from build123d import *

# Parameters (mm, degrees)
CYLINDER002_R     = 35
CYLINDER002_DEPTH = 50
CYLINDER001_R     = 35
CYLINDER001_DEPTH = 50
BOX001_W          = 102
BOX001_H          = 260
BOX001_DEPTH      = 50
CYLINDER_R        = 37
CYLINDER_DEPTH    = 45
CYLINDER003_R     = 37
CYLINDER003_DEPTH = 45
BOX_W             = 40
BOX_H             = 270
BOX_DEPTH         = 25
CHAMFER_SIZE      = 1.5


with BuildPart() as cylinder002:
    # Cylinder002 → Cylinder002 (new body)
    with BuildSketch(Plane(origin=(40, 230, -45), x_dir=(1, 0, 0), z_dir=(0, 0, 1))):
        Circle(CYLINDER002_R)
    extrude(amount=CYLINDER002_DEPTH)


with BuildPart() as cylinder001:
    # Cylinder001 → Cylinder001 (new body)
    with BuildSketch(Plane(origin=(40, 40, -45), x_dir=(1, 0, 0), z_dir=(0, 0, 1))):
        Circle(CYLINDER001_R)
    extrude(amount=CYLINDER001_DEPTH)


with BuildPart() as main_cutout:
    # Box001 → Box001 (new body)
    with BuildSketch(Plane(origin=(5, 5, 5), x_dir=(1, 0, 0), z_dir=(0, 0, 1))):
        with Locations((51, 130)):
            Rectangle(BOX001_W, BOX001_H)
    extrude(amount=BOX001_DEPTH)


with BuildPart() as cylinder:
    # Cylinder → Cylinder (new body)
    with BuildSketch(Plane(origin=(40, 40, -20), x_dir=(1, 0, 0), z_dir=(0, 0, 1))):
        Circle(CYLINDER_R)
    extrude(amount=CYLINDER_DEPTH)


with BuildPart() as cylinder003:
    # Cylinder003 → Cylinder003 (new body)
    with BuildSketch(Plane(origin=(40, 230, -20), x_dir=(1, 0, 0), z_dir=(0, 0, 1))):
        Circle(CYLINDER003_R)
    extrude(amount=CYLINDER003_DEPTH)


with BuildPart() as chamfer_body:
    # Box → Box (new body)
    with BuildSketch(Plane.XY):
        with Locations((20, 135)):
            Rectangle(BOX_W, BOX_H)
    extrude(amount=BOX_DEPTH)

    # Fusion: union Cylinder, Cylinder003
    add(cylinder.part)
    add(cylinder003.part)

    # Cut: cut Main cutout
    add(main_cutout.part, mode=Mode.SUBTRACT)

    # Cut001: cut Cylinder001
    add(cylinder001.part, mode=Mode.SUBTRACT)

    # Cut002: cut Cylinder002
    add(cylinder002.part, mode=Mode.SUBTRACT)

    # Chamfer
    chamfer_edges = [chamfer_body.edges().sort_by_distance(p)[0] for p in [
        (40, 0, 12.5),
        (40, 270, 12.5),
    ]]
    chamfer(chamfer_edges, length=CHAMFER_SIZE)


solid = chamfer_body.part
Part model, mm, in its own coordinate system. A direction names the side the tool comes from. Give positions to 0.01 mm unless a question says otherwise; leave off trailing zeros. Order: outer loops, then holes, each group sorted by start corner. A loop starts at its lowest first (then second) coordinate and runs counter-clockwise, first axis right, second up. Notation, with made-up numbers: (56, -27.5) -> (83, -27.5) arc R22 ccw to (83, -3.5) -> close; hole circle Ø8 at (71.25, -32). An arc over 180 degrees is marked (long way). Use one line per item in the form item = value.
(1) Saw through at A-A (z = 18). Write the cut outline in (x, y), then the cut area to 3 significant figures.
Solution:
outline = (0, 0) -> (38.5, 0) -> (40, 1.5) -> (40, 3) arc R37 ccw to (52, 5) -> (5, 5) -> (5, 265) -> (52, 265) arc R37 ccw to (40, 267) -> (40, 268.5) -> (38.5, 270) -> (0, 270) -> close
area = 1,730 mm²
(2) Saw through at B-B (x = 17.5). Write the cut outline in (y, z), then the cut area to 3 significant figures.
Solution:
outline = (0, 0) -> (10.63, 0) -> (10.63, -20) -> (13.19, -20) -> (13.19, 5) -> (5, 5) -> (5, 25) -> (0, 25) -> close; (66.81, -20) -> (69.37, -20) -> (69.37, 0) -> (200.63, 0) -> (200.63, -20) -> (203.19, -20) -> (203.19, 5) -> (66.81, 5) -> close; (256.81, -20) -> (259.37, -20) -> (259.37, 0) -> (270, 0) -> (270, 25) -> (265, 25) -> (265, 5) -> (256.81, 5) -> close
area = 1,220 mm²
(3) Saw through at D-D (z = -9). Write the cut outline in (x, y), then the cut area to 3 significant figures.
Solution:
outline = circle Ø74 at (40, 40); circle Ø74 at (40, 230); hole circle Ø70 at (40, 40); hole circle Ø70 at (40, 230)
area = 905 mm²
(4) Tool access for faces 5 (the face through (15, 137, 0)), 6 (the face through (25, 136, 5)), 7 (the face through (74.18, 25.83, -7.81)), 8 (the face through (4.7, 165.6, 25)): list every direction of +Z, -Z, +X, -X, +Y, -Y with a clear straight run to the whole face (end or side of a thin tool).
Solution:
face_5 = -Z, -X
face_6 = +Z, +X
face_7 = -Z
face_8 = +Z, +X, -X, +Y, -Y
(5) Flat gauge pins, fed straight in: P1, Ø2, axis at y = 97, z = -0.5, coming from the +X side; P2, Ø12, axis at x = 45.5, z = 0, coming from the +Y side; P3, Ø5, axis at y = 136, z = 10, coming from the +X side; P4, Ø1, axis at x = 60, y = 72, coming from the +Z side. Where does each tip first touch, or does it go through?
Solution:
P1 = 40
P2 = 269
P3 = 5
P4 = through
(6) Saw through at C-C (y = 208). Write the cut outline in (x, z).
Solution:
outline = (0, 0) -> (10.25, 0) -> (10.25, -20) -> (12.78, -20) -> (12.78, 5) -> (5, 5) -> (5, 25) -> (0, 25) -> close; (67.22, -20) -> (69.75, -20) -> (69.75, 5) -> (67.22, 5) -> close
(7) Pull direction Y, two halves, no side cores. Call faces 1 (the face through (19, 270, 12)), 2 (the face through (0, 133, 12)), 3 (the face through (35.44, 264.7, -7.67)), 4 (the face through (40, 134, 2)): +Y half, -Y half, draft (parallel to the pull), parting line (faces both ways), or undercut.
Solution:
face_1 = +Y half
face_2 = draft
face_3 = undercut
face_4 = undercut
(8) Drill centre lines: line 1 (Y direction, x = 40, z = -3); line 2 (X direction, y = 230, z = -7.25); line 3 (Y direction, x = 18, z = 9). Where is each one in solid material? Low to high. Write a range as from..to.
Solution:
line_1 = 3..5, 75..77, 193..195, 265..267
line_2 = 3..5, 75..77
line_3 = 0..5, 265..270
